from build123d import *

# Parameters (mm, degrees)
SKETCH1_W           = 110
SKETCH1_H           = 90
BOSS_EXTRUDE2_DEPTH = 27.5
CUT_EXTRUDE5_DEPTH  = 90
SKETCH5_R           = 1.5
CUT_EXTRUDE7_DEPTH  = 7.5
SKETCH7_R           = 1.5
CUT_EXTRUDE9_DEPTH  = 7.5
SKETCH9_R           = 1.5
CUT_EXTRUDE11_DEPTH = 7.5
SKETCH12_R          = 1.5
CUT_EXTRUDE14_DEPTH = 7.5
CUT_EXTRUDE22_DEPTH = 2
SKETCH18_5_W        = 3
SKETCH18_5_H        = 12
CUT_EXTRUDE23_DEPTH = 5
SKETCH23_R          = 2
SKETCH23_R_2        = 4
CUT_EXTRUDE24_DEPTH = 5
SKETCH24_R          = 4
CUT_EXTRUDE25_DEPTH = 5
SKETCH25_W          = 15
SKETCH25_H          = 8
CUT_EXTRUDE26_DEPTH = 5


with BuildPart() as part:
    # Sketch1 → Boss-Extrude2 (new body)
    with BuildSketch(Plane(origin=(0, 0, 0), x_dir=(1, 0, 0), z_dir=(0, 1, 0))):
        Rectangle(SKETCH1_W, SKETCH1_H)
    extrude(amount=BOSS_EXTRUDE2_DEPTH)

    # Sketch4 → Cut-Extrude5 (cut)
    with BuildSketch(Plane.XY.offset(45)):
        Polygon((50, 2.5), (-50, 21.547619048), (-50, 20), (-55, 20), (-55, 0), (50, 0), align=None)
        Polygon((-50, 27.5), (-50, 26.547619048), (50, 7.5), (55, 7.5), (55, 27.5), align=None)
        Polygon((-50, 27.5), (-55, 27.5), (-50, 26.547619048), align=None)
        Polygon((-50, 26.547619048), (-55, 27.5), (-55, 26.547619048), align=None)
    extrude(amount=-CUT_EXTRUDE5_DEPTH, mode=Mode.SUBTRACT)

    # Sketch5 → Cut-Extrude7 (cut)
    with BuildSketch(Plane(origin=(0, 7.5, 0), x_dir=(1, 0, 0), z_dir=(0, 1, 0))):
        with Locations((52.5, 42.5)):
            Circle(SKETCH5_R)
    extrude(amount=-CUT_EXTRUDE7_DEPTH, mode=Mode.SUBTRACT)

    # Sketch7 → Cut-Extrude9 (cut)
    with BuildSketch(Plane(origin=(0, 7.5, 0), x_dir=(1, 0, 0), z_dir=(0, 1, 0))):
        with Locations((52.5, -42.5)):
            Circle(SKETCH7_R)
    extrude(amount=-CUT_EXTRUDE9_DEPTH, mode=Mode.SUBTRACT)

    # Sketch9 → Cut-Extrude11 (cut)
    with BuildSketch(Plane(origin=(0, 26.547619048, 0), x_dir=(1, 0, 0), z_dir=(0, 1, 0))):
        with Locations((-52.5, 42.5)):
            Circle(SKETCH9_R)
    extrude(amount=-CUT_EXTRUDE11_DEPTH, mode=Mode.SUBTRACT)

    # Sketch12 → Cut-Extrude14 (cut)
    with BuildSketch(Plane(origin=(0, 26.547619048, 0), x_dir=(1, 0, 0), z_dir=(0, 1, 0))):
        with Locations((-52.5, -42.5)):
            Circle(SKETCH12_R)
    extrude(amount=-CUT_EXTRUDE14_DEPTH, mode=Mode.SUBTRACT)

    # Sketch18 → Cut-Extrude22 (cut)
    with BuildSketch(Plane(origin=(3.129102845, 16.427789934, 0), x_dir=(0.982338566, -0.187112108, 0), z_dir=(0.187112108, 0.982338566, 0))):
        Polygon((9.356793756, -6), (6.356793756, -6), (6.356793756, -18.5), (41.356793756, -18.5), (41.356793756, 18.5), (6.356793756, 18.5), (6.356793756, 6), (9.356793756, 6), align=None)
    extrude(amount=-CUT_EXTRUDE22_DEPTH, mode=Mode.SUBTRACT)

    # Sketch18_5 → Cut-Extrude23 (cut)
    with BuildSketch(Plane(origin=(3.129102845, 16.427789934, 0), x_dir=(0.982338566, -0.187112108, 0), z_dir=(0.187112108, 0.982338566, 0))):
        with Locations((7.856793756, 0)):
            Rectangle(SKETCH18_5_W, SKETCH18_5_H)
    extrude(amount=-CUT_EXTRUDE23_DEPTH, mode=Mode.SUBTRACT)

    # Sketch23 → Cut-Extrude24 (cut)
    with BuildSketch(Plane(origin=(3.129102845, 16.427789934, 0), x_dir=(0.982338566, -0.187112108, 0), z_dir=(0.187112108, 0.982338566, 0))):
        with Locations((-41.584309281, -33)):
            Circle(SKETCH23_R)
        with Locations((-27.584309281, -33)):
            Circle(SKETCH23_R)
        with Locations((-36.584309281, -27)):
            Circle(SKETCH23_R_2)
    extrude(amount=-CUT_EXTRUDE24_DEPTH, mode=Mode.SUBTRACT)

    # Sketch24 → Cut-Extrude25 (cut)
    with BuildSketch(Plane(origin=(3.129102845, 16.427789934, 0), x_dir=(0.982338566, -0.187112108, 0), z_dir=(0.187112108, 0.982338566, 0))):
        with Locations((22.713587512, -30)):
            Circle(SKETCH24_R)
    extrude(amount=-CUT_EXTRUDE25_DEPTH, mode=Mode.SUBTRACT)

    # Sketch25 → Cut-Extrude26 (cut)
    with BuildSketch(Plane(origin=(3.129102845, 16.427789934, 0), x_dir=(0.982338566, -0.187112108, 0), z_dir=(0.187112108, 0.982338566, 0))):
        with Locations((30.213587512, 31.5)):
            Rectangle(SKETCH25_W, SKETCH25_H)
    extrude(amount=-CUT_EXTRUDE26_DEPTH, mode=Mode.SUBTRACT)


solid = part.part
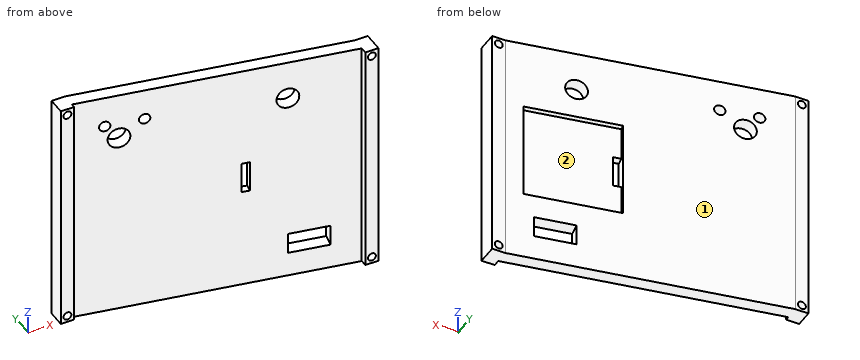
The listing builds one solid part. Answer for the finished solid, in the listing's coordinates (mm). Face numbers are marked on the shaded views. Round coordinates to 2 decimals unless told otherwise and drop trailing zeros. Write each loop counter-clockwise with the first axis right and the second up, starting at its lowest first coordinate (ties: lowest second). Pieces come first, ordered by that corner, then holes. Notation, with made-up numbers: M -10.75,32.25 L 29.25,32.25 A17 ccw 29.25,65.25 Z; hole C 54.25,31 d7. An arc over 180 degrees is marked long. Write each question's results on one line, items separated by ' | '. Start each with the question number.
(1) Determine the mould class of the marked faces 1 and 2 for opening direction X: +X half, -X half, draft (parallel to the pull), parting line (faces both ways), or undercut.
(2) The part is cut by section A-A, the plane x = -52.5. Write down the section's boundary in (y, z), and give its area (3 significant figures).
(3) The part is cut by section C-C, the plane z = -25.5. Write down the section's boundary in (x, y).
(4) Find the intervals of material crossed by line 1 (Z direction, x = 52.5, y = 1.5); line 2 (Y direction, x = 41, z = 19); line 3 (Y direction, x = 46, z = 22.5), in increasing order.
(5) The part is cut by section D-D, the plane x = 52.5. Write down the section's boundary in (y, z), and give its area (3 significant figures).
(6) The part is cut by section B-B, the plane z = -42.5. Write down the section's boundary in (x, y).
(7) Each of these flat-tipped pins is pushed along its axis until it touches: P1, Ø6, axis at x = 38, z = 5, coming from the +Y side; P2, Ø4, axis at x = 2.5, y = 8, coming from the +Z side; P3, Ø4, axis at x = 52.5, z = 42.5, coming from the +Y side; P4, Ø1.5, axis at x = -31.5, z = -25, coming from the +Y side. Where does it stop, or does it pass through?
Worked answers:
1) face 1: +X half | face 2: undercut
2) outline: M 20,-45 L 26.55,-45 L 26.55,-44 L 20,-44 Z; M 20,-41 L 26.55,-41 L 26.55,41 L 20,41 Z; M 20,44 L 26.55,44 L 26.55,45 L 20,45 Z | area: 550 mm²
3) outline: M -55,20 L -50,20 L -50,21.55 L 50,2.5 L 50,0 L 55,0 L 55,7.5 L 50,7.5 L -50,26.55 L -55,26.55 Z
4) line 1: z = -45 to -44, -41 to 41, 44 to 45 | line 2: y = 4.21 to 9.21 | line 3: y = 3.26 to 8.26
5) outline: M 0,-45 L 7.5,-45 L 7.5,-44 L 0,-44 Z; M 0,-41 L 7.5,-41 L 7.5,41 L 0,41 Z; M 0,44 L 7.5,44 L 7.5,45 L 0,45 Z | area: 630 mm²
6) outline: M -55,20 L -54,20 L -54,26.55 L -55,26.55 Z; M -51,20 L -50,20 L -50,21.55 L 50,2.5 L 50,0 L 51,0 L 51,7.5 L 50,7.5 L -50,26.55 L -51,26.55 Z; M 54,0 L 55,0 L 55,7.5 L 54,7.5 Z
7) P1: stops at y = 8.32 | P2: passes through | P3: stops at y = 7.5 | P4: stops at y = 23.17
